For this review, use the dimensioned drawing (mm, ordinates from the lowest corner) and the shaded views. Coordinates: 2 decimals unless noted, no trailing zeros. Write each loop counter-clockwise with the first axis right and the second up, starting at its lowest first coordinate (ties: lowest second). Pieces come first, ordered by that corner, then holes. Notation, with made-up numbers: (55, -28.75) - (98, -28.75) arc R18 cw to (98, -14.75) - close; hole circle Ø1 at (71.5, 70). An arc over 180 degrees is marked (long way). One line per item, written item: value.
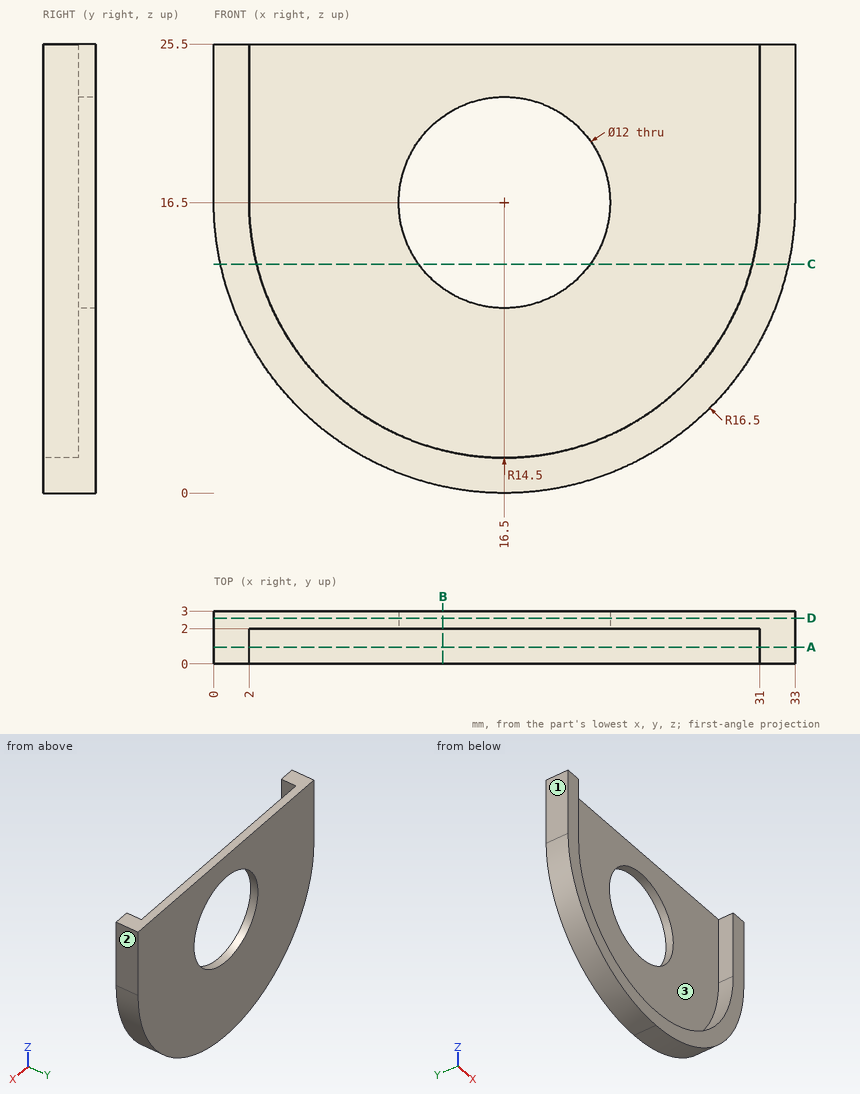
1. Consider section C-C, the plane z = 13. Write out the cut boundary in (x, y), then the cut area to 3 significant figures.
Answer block:
outline: (0.38, 0) - (2.43, 0) - (2.43, 2) - (11.63, 2) - (11.63, 3) - (0.38, 3) - close; (21.37, 2) - (30.57, 2) - (30.57, 0) - (32.62, 0) - (32.62, 3) - (21.37, 3) - close
area: 30.7 mm^2
2. Consider section D-D, the plane y = 2.6. Write out the cut boundary in (x, z), then the cut area to 3 significant figures.
Answer block:
outline: (0, 16.5) arc R16.5 ccw to (33, 16.5) - (33, 25.5) - (0, 25.5) - close; hole circle Ø12 at (16.5, 16.5)
area: 612 mm^2
3. Consider section B-B, the plane x = 13. Write out the cut boundary in (y, z), then the cut area to 3 significant figures.
Answer block:
outline: (0, 0.38) - (3, 0.38) - (3, 11.63) - (2, 11.63) - (2, 2.43) - (0, 2.43) - close; (2, 21.37) - (3, 21.37) - (3, 25.5) - (2, 25.5) - close
area: 19.5 mm^2
4. Wall thickness on line 1 along X through (y, z) = (1.95, 20.25); line 2 along X through (y, z) = (2.25, 16.5); line 3 along Y through (x, z) = (23, 6.75): over which ranges is each line inside the solid? List them lowest first.
Answer block:
line 1: x = 0 to 2, 31 to 33
line 2: x = 0 to 10.5, 22.5 to 33
line 3: y = 2 to 3
5. Consider section A-A, the plane y = 0.95. Write out the cut boundary in (x, z), then the cut area to 3 significant figures.
Answer block:
outline: (0, 16.5) arc R16.5 ccw to (33, 16.5) - (33, 25.5) - (31, 25.5) - (31, 16.5) arc R14.5 cw to (2, 16.5) - (2, 25.5) - (0, 25.5) - close
area: 133 mm^2
6. Insertion check: pin 1 Ø1.5 at (x, z) = (24, 17.5) entering from -Y; pin 2 Ø7 at (x, z) = (16.5, 16.5) entering from +Y; pin 3 Ø1.5 at (x, y) = (17.5, 2) entering from -Z. Each pin has a flat end and moves straight along its axis. Give the tip position at first contact, or say it passes through.
Answer block:
pin 1: stops at y = 2
pin 2: passes through
pin 3: stops at z = 0
7. Mouldability with a two-part tool opening along X and no side actions: class the marked faces 1, 2 and 3 as released by +X, released by -X, zero draft, split by the parting line, or undercut.
Answer block:
face 1: released by -X
face 2: released by +X
face 3: undercut
